```python
from build123d import *

# Parameters (mm, degrees)
F2_R     = 3.96875
F3_DEPTH = 9.525
F4_R     = 1.5875
F5_DEPTH = 20.6375


# Not quite as in the source:
# - a length typed as a fraction of an inch, garbled in the dataset ("3 / 203.2 mm" for 3/8 in), is restored


with BuildPart() as f1:
    # F0 (on Front) → F1 (revolve)
    with BuildSketch(Plane.XZ):
        with BuildLine():
            Line((0, 30.1625), (0, 0))
            Line((0, 0), (5.2339527756, 0))
            ThreePointArc((5.2339527756, 0), (6.9300739719, 1.2963017107), (7.94385, 3.17499365))
            Line((7.94385, 3.17499365), (7.9375, 6.3499873))
            Line((7.9375, 6.3499873), (25.0110084837, 6.3499873))
            ThreePointArc((25.0110084837, 6.3499873), (31.8322699863, 8.6224170081), (25.0874177301, 11.1125))
            Line((25.0874177301, 11.1125), (7.9375, 11.1125))
            Line((7.9375, 11.1125), (7.9375, 28.8007091731))
            ThreePointArc((7.9375, 28.8007091731), (7.6114687199, 29.8820156927), (6.517462898, 30.1625))
            Line((6.517462898, 30.1625), (0, 30.1625))
        make_face()
    revolve(axis=Axis((0, 0, 15.08125), (0, 0, 1)))

    # F2 (on face) → F3 (cut)
    with BuildSketch(Plane.XY.offset(30.1625)):
        Circle(F2_R)
    extrude(amount=-F3_DEPTH, mode=Mode.SUBTRACT)

    # F4 (on face) → F5 (cut)
    with BuildSketch(Plane(origin=(0, 0, 0), x_dir=(1, 0, 0), z_dir=(0, 0, -1))):
        Circle(F4_R)
    extrude(amount=-F5_DEPTH, mode=Mode.SUBTRACT)


solid = f1.part
```
Source: CAD feature listing. Evaluate the final solid. Frame: model axes, mm. Coordinates: 2 decimals unless noted, no trailing zeros. Order: outer loops, then holes, each group sorted by start corner. A loop starts at its lowest first (then second) coordinate and runs counter-clockwise, first axis right, second up. Notation, with made-up numbers: M 69.5,36.25 L 107.5,36.25 A22 ccw 107.5,67.25 Z; hole C 39,24.25 d2. An arc over 180 degrees is marked long. Write each question's results on one line, items separated by ' | '. Start each with the question number.
1) Line query: line 1 (X direction, y = 14.5, z = 5.5); line 2 (Z direction, x = -9, y = 9.5); line 3 (X direction, y = 1.5, z = 28.5). Output: solid intervals per line, ascending. Write a range as from..to.
2) Section query B-B (z = 18). Return the cut outline in (x, y) (1 decimal), plus the area to 3 significant figures.
3) Contact query for flat-ended pins moving along their axis: pin 1 Ø1 at (y, z) = (9, 20) entering from -X; pin 2 Ø3 at (y, z) = (-0.5, 22) entering from -X; pin 3 Ø8 at (x, z) = (2, 26.5) entering from +Y; pin 4 Ø2.5 at (x, y) = (0, 1) entering from +Z. Output: stop coordinate, or through.
4) Section query A-A (z = 28). Return the cut outline in (x, y) (1 decimal).
5) Draft query along Y for faces 1 (the face through (1.24, 1.24, 0)), 2 (the face through (-0.34, 1.55, 10.17)). Return one class per face: released by +Y, released by -Y, zero draft, split by the parting line, or undercut.
Answers:
1) line 1: x = -26.4..-21.5, 21.5..26.4 | line 2: z = 6.35..11.11 | line 3: x = -7.79..-3.67, 3.67..7.79
2) outline: C 0,0 d15.9; hole C 0,0 d3.2 | area: 190 mm^2
3) pin 1: passes through | pin 2: stops at x = -7.94 | pin 3: stops at y = 7.97 | pin 4: stops at z = 20.64
4) outline: C 0,0 d15.9; hole C 0,0 d7.9
5) face 1: zero draft | face 2: undercut
